Check sheet for the drawn part. Datum: minimum x, y, z corner. Units: mm. A direction names the side the tool comes from. Round coordinates to 2 decimals unless told otherwise and drop trailing zeros. Loops run counter-clockwise (first coordinate to the right, second up) from the corner with the lowest first, then second, coordinate; pieces in that order, holes last. Notation, with made-up numbers: (25, -28) -> (43, -28) arc R25 ccw to (43, -8) -> close; hole circle Ø3 at (55, 55). An arc over 180 degrees is marked (long way). Return JSON: item names as keys, results as strings.
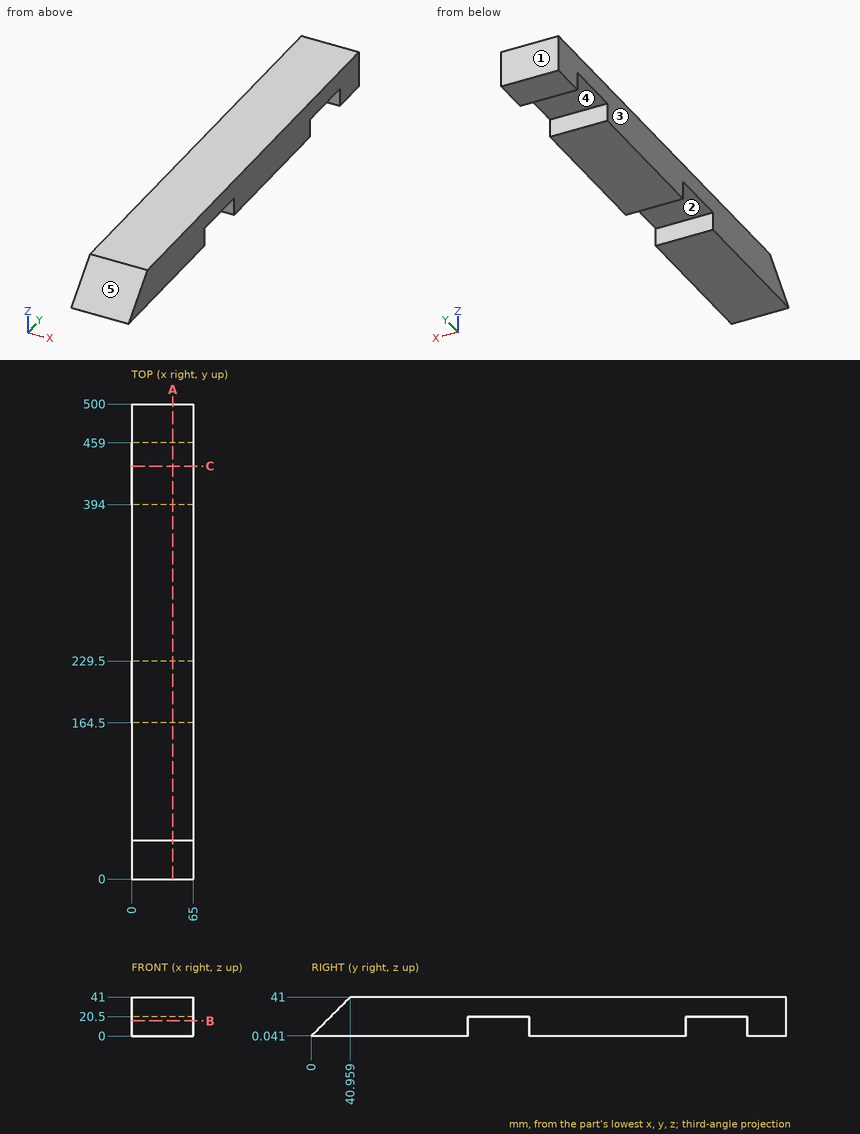
Q1. Material ranges on line 1 (Y direction, x = 44, z = 12); line 2 (Y direction, x = 28, z = 20); line 3 (Z direction, x = 39, y = 434), recorded low to high.
Results list:
{"line 1": "11.96 to 164.5, 229.5 to 394, 459 to 500", "line 2": "19.96 to 164.5, 229.5 to 394, 459 to 500", "line 3": "20.5 to 41"}
Q2. Go/stop test with flat-tipped pins: pin 1 (1 mm diameter, centred on x = 57.5, z = 4.5, fed in from -Y); pin 2 (10 mm diameter, centred on x = 25, z = 6, fed in from -Y); pin 3 (2 mm diameter, centred on x = 11, y = 206.5, fed in from -Z). Record where each tip stops, or that it passes through.
Results list:
{"pin 1": "y = 3.96", "pin 2": "y = 0.96", "pin 3": "z = 20.5"}
Q3. Section check B-B (z = 16). Record the boundary of the cut face in (x, y).
Results list:
{"outline": "(0, 15.96) -> (65, 15.96) -> (65, 164.5) -> (0, 164.5) -> close; (0, 229.5) -> (65, 229.5) -> (65, 394) -> (0, 394) -> close; (0, 459) -> (65, 459) -> (65, 500) -> (0, 500) -> close"}
Q4. Tool access check on the marked faces 4 and 5. Record the directions out of +Z, -Z, +X, -X, +Y, -Y that give a thin tool (end or side, any length) a straight path to the whole face; none if there is none.
Results list:
{"face 4": "-Z, +X, -X", "face 5": "+Z, +X, -X, -Y"}
Q5. Draft check along Y on the marked faces 1, 2 and 3. Enter one of: released by +Y, released by -Y, zero draft, split by the parting line, or undercut.
Results list:
{"face 1": "released by +Y", "face 2": "undercut", "face 3": "zero draft"}
Q6. Section check C-C (y = 434.5). Record the boundary of the cut face in (x, z), then the cut area to 3 significant figures.
Results list:
{"outline": "(0, 20.5) -> (65, 20.5) -> (65, 41) -> (0, 41) -> close", "area": "1,330 mm^2"}
Q7. Section check A-A (x = 43.5). Record the boundary of the cut face in (y, z), then the cut area to 3 significant figures.
Results list:
{"outline": "(0, 0) -> (164.5, 0) -> (164.5, 20.5) -> (229.5, 20.5) -> (229.5, 0) -> (394, 0) -> (394, 20.5) -> (459, 20.5) -> (459, 0) -> (500, 0) -> (500, 41) -> (40.96, 41) -> (0, 0.04) -> close", "area": "17,000 mm^2"}
